Drawing for the job (mm, zero at the part's lowest x, y, z). Give positions to 0.01 mm unless a question says otherwise; leave off trailing zeros. Loops run counter-clockwise (first coordinate to the right, second up) from the corner with the lowest first, then second, coordinate; pieces in that order, holes last. Notation, with made-up numbers: (-7, 77) -> (-3, 77) arc R20 ccw to (-3, 100) -> close; hole circle Ø2 at (15, -17). An arc over 180 degrees is marked (long way). Use CSV: the item, a comma, the result in double quotes. Start each with the question number.
(1) Drill centre lines: probe 1 along Z at (x, y) = (48, 10.5); probe 2 along Y at (x, z) = (28.5, 9); probe 3 along X at (y, z) = (16, 27). Where is each one in solid material? Low to high.
(2) Cut at A-A on z = 26. Write the cut outline in (x, y), then the cut area to 3 significant figures.
(3) Cut at B-B on x = 48. Write the cut outline in (y, z).
(4) Flat gauge pins, fed straight in: pin 1 (8 mm diameter, centred on x = 62, z = 3, fed in from -Y); pin 2 (2 mm diameter, centred on x = 116.5, y = 2, fed in from -Z); pin 3 (5 mm diameter, centred on x = 152, z = 26, fed in from -Y). Where does each tip first touch, or does it go through?
(5) Cut at C-C on y = 18.5. Write the cut outline in (x, z), then the cut area to 3 significant figures.
(6) Cut at D-D on z = 7.5. Write the cut outline in (x, y), then the cut area to 3 significant figures.
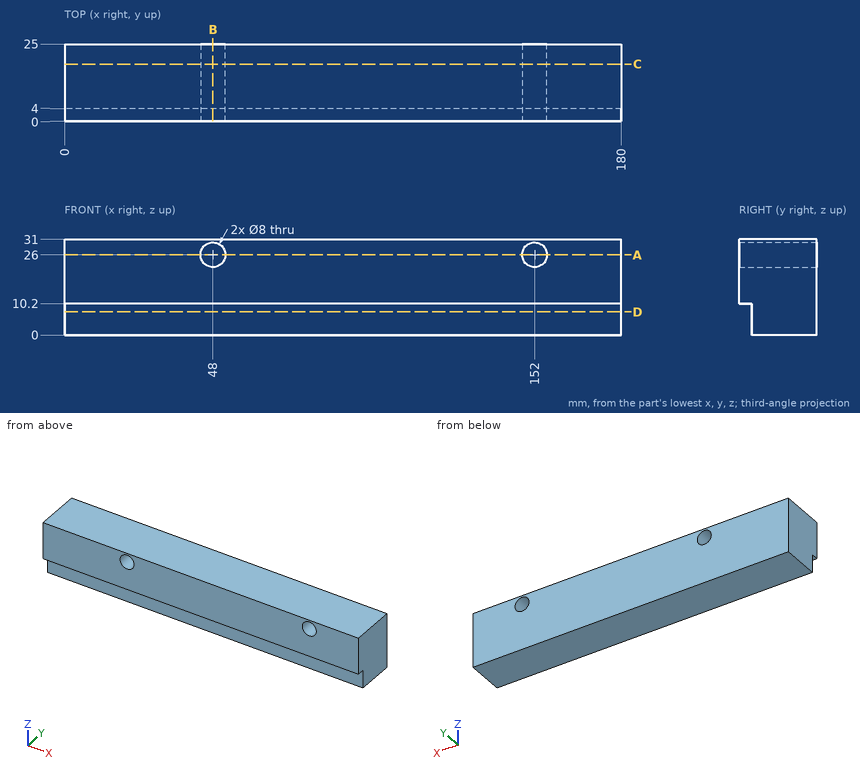
Check result:
1,probe 1,"0 to 22, 30 to 31"
1,probe 2,"4 to 25"
1,probe 3,"0 to 44.13, 51.87 to 148.13, 155.87 to 180"
2,outline,"(0, 0) -> (44, 0) -> (44, 25) -> (0, 25) -> close; (52, 0) -> (148, 0) -> (148, 25) -> (52, 25) -> close; (156, 0) -> (180, 0) -> (180, 25) -> (156, 25) -> close"
2,area,"4,100 mm²"
3,outline,"(0, 10.2) -> (4, 10.2) -> (4, 0) -> (25, 0) -> (25, 22) -> (0, 22) -> close; (0, 30) -> (25, 30) -> (25, 31) -> (0, 31) -> close"
4,pin 1,"y = 4"
4,pin 2,"z = 10.2"
4,pin 3,"through"
5,outline,"(0, 0) -> (180, 0) -> (180, 31) -> (0, 31) -> close; hole circle Ø8 at (48, 26); hole circle Ø8 at (152, 26)"
5,area,"5,480 mm²"
6,outline,"(0, 4) -> (180, 4) -> (180, 25) -> (0, 25) -> close"
6,area,"3,780 mm²"
